```python
from build123d import *

# Parameters (mm, degrees)
F0_R     = 37.3678316612
F0_R_2   = 36.1312756735
F1_DEPTH = 90
F2_R     = 1


# Not quite as in the source:
# - a fillet or chamfer that OpenCascade refuses, or shapes differently, is made with other operations: its cross-section is extruded or revolved along the edge and cut away or added


with BuildPart() as f1:
    # F0 (on Front) → F1 (new body)
    with BuildSketch(Plane.XZ):
        Circle(F0_R)
        Circle(F0_R_2, mode=Mode.SUBTRACT)
    extrude(amount=F1_DEPTH)

    # F2
    f2_edges = [f1.edges().sort_by_distance(p)[0] for p in [
        (37.367832, -45, 0),
        (-37.367832, 0, 0),
        (-37.367832, -90, 0),
    ]]
    fillet(f2_edges, radius=F2_R)

    # F3: chamfer of 1 on 2 edges, made by hand

    # F3_s1 → F3_t2 (revolve, cut)
    with BuildSketch(Plane.XY):
        Polygon((37.1312756735, -90), (36.1312756735, -89), (36.1312756735, -90), align=None)
    revolve(axis=Axis((0, -90, 0), (0, -1, 0)), mode=Mode.SUBTRACT)


solid = f1.part
```
Geometry: final body of the model. Coordinates: model frame, mm. Coordinates: 2 decimals unless noted, no trailing zeros. Write each loop counter-clockwise with the first axis right and the second up, starting at its lowest first coordinate (ties: lowest second). Pieces come first, ordered by that corner, then holes. Notation, with made-up numbers: M 11,44.25 L 37,44.25 A22 ccw 37,69.25 Z; hole C -19.75,-37 d4. An arc over 180 degrees is marked long. Use CSV: the item, a comma, the result in double quotes. Start each with the question number.
1. Cut plane C-C on y = -52. Return the cut outline in (x, z).
2. Ray query, probe 1 along Z at (x, y) = (0, -64); probe 2 along Z at (x, y) = (14, -70); probe 3 along X at (y, z) = (-5, -11.5). Return the intervals inside material, ascending.
3. Cut plane B-B on x = 0. Return the cut outline in (y, z), plus the area to 3 significant figures.
4. Cut plane A-A on z = 0. Return the cut outline in (x, y).
5. First-contact query: P1, Ø3, axis at y = -29.5, z = 2.5, coming from the -X side; P2, Ø1, axis at x = 20, y = -25.5, coming from the +Z side; P3, Ø1.5, axis at y = -13, z = 3.5, coming from the +X side. Flat tips, straight axial feed; report the tip coordinate or a pass-through.
6. Mould query, pull axis Z, two halves, no side actions, for faces 1 (the face through (34.52, -44.38, -14.31)), 2 (the face through (-28.67, -43.88, -21.99)). Classes: pulls with the +Z half, pulls with the -Z half, needs draft (parallel to the pull), parting line crosses it, or undercut.
Entries:
1,outline,"C 0,0 d74.74; hole C 0,0 d72.26"
2,probe 1,"-37.37 to -36.13, 36.13 to 37.37"
2,probe 2,"-34.65 to -33.31, 33.31 to 34.65"
2,probe 3,"-35.55 to -34.25, 34.25 to 35.55"
3,outline,"M -89.82,-36.95 A1 ccw -89,-37.37 L -1,-37.37 A1 ccw 0,-36.37 L 0,-36.13 L -89,-36.13 Z; M -89.82,36.95 L -89,36.13 L 0,36.13 L 0,36.37 A1 ccw -1,37.37 L -89,37.37 A1 ccw Z"
3,area,"221 mm²"
4,outline,"M -37.37,-89 A1 ccw -36.95,-89.82 L -36.13,-89 L -36.13,0 L -36.37,0 A1 ccw -37.37,-1 Z; M 36.13,-89 L 36.95,-89.82 A1 ccw 37.37,-89 L 37.37,-1 A1 ccw 36.37,0 L 36.13,0 Z"
5,P1,"x = -37.35"
5,P2,"z = 31.88"
5,P3,"x = 37.27"
6,face 1,"parting line crosses it"
6,face 2,"undercut"
